Verification items for the finished model (mm, model axes). Face numbers are marked on the shaded views. A direction names the side the tool comes from. Give positions to 0.01 mm unless a question says otherwise; leave off trailing zeros. Order: outer loops, then holes, each group sorted by start corner. A loop starts at its lowest first (then second) coordinate and runs counter-clockwise, first axis right, second up. Notation, with made-up numbers: (65.5, -10.5) - (119.5, -10.5) arc R22 cw to (119.5, -0.5) - close; hole circle Ø11 at (25, -35). An arc over 180 degrees is marked (long way). Answer as a JSON object with one key per item and string values.
```python
from build123d import *

# Parameters (mm, degrees)
SKETCH1_W                    = 22.7711
SKETCH1_H                    = 12.18
BOSS_EXTRUDE1_DEPTH          = 23.79
SKETCH3_W                    = 32.4485
SKETCH3_H                    = 12.18
BOSS_EXTRUDE2_DEPTH          = 2.286
CUT_EXTRUDE1_DEPTH           = 36.695245613
BOSS_EXTRUDE3_DEPTH          = 4.3434
SKETCH6_R                    = 2.3495
BOSS_EXTRUDE4_DEPTH          = 2.7813
SKETCH7_W                    = 2.8956
SKETCH7_H                    = 1.0414
BOSS_EXTRUDE5_DEPTH          = 6.096
M2_5X0_45_TAPPED_HOLE1_D     = 2.05
M2_5X0_45_TAPPED_HOLE1_DEPTH = 4
M2_5X0_45_TAPPED_HOLE1_TIP   = 0.615882135


with BuildPart() as part:
    # Sketch1 → Boss-Extrude1 (new body)
    with BuildSketch(Plane(origin=(0, 0, 0), x_dir=(1, 0, 0), z_dir=(0, 1, 0))):
        with Locations((11.38555, 6.09)):
            Rectangle(SKETCH1_W, SKETCH1_H)
    extrude(amount=BOSS_EXTRUDE1_DEPTH)

    # Sketch3 → Boss-Extrude2 (add)
    with BuildSketch(Plane(origin=(0, 19.0656, 0), x_dir=(1, 0, 0), z_dir=(0, 1, 0))):
        with Locations((11.38555, 6.09)):
            Rectangle(SKETCH3_W, SKETCH3_H)
    extrude(amount=-BOSS_EXTRUDE2_DEPTH)

    # Sketch4 → Cut-Extrude1 (cut, through all)
    with BuildSketch(Plane(origin=(0, 19.0656, 0), x_dir=(1, 0, 0), z_dir=(0, 1, 0))):
        with BuildLine():
            Line((-4.8387, 6.6996), (-3.4671, 6.6996))
            ThreePointArc((-3.4671, 6.6996), (-1.6383, 6.09), (-3.4671, 5.4804))
            Line((-3.4671, 5.4804), (-4.8387, 5.4804))
            Line((-4.8387, 5.4804), (-4.8387, 6.6996))
        make_face()
        with BuildLine():
            Line((26.2382, 5.4804), (27.6098, 5.4804))
            Line((27.6098, 5.4804), (27.6098, 6.6996))
            Line((27.6098, 6.6996), (26.2382, 6.6996))
            ThreePointArc((26.2382, 6.6996), (24.4094, 6.09), (26.2382, 5.4804))
        make_face()
    extrude(amount=-CUT_EXTRUDE1_DEPTH, mode=Mode.SUBTRACT)

    # Sketch5 → Boss-Extrude3 (add)
    with BuildSketch(Plane(origin=(0, 23.79, 0), x_dir=(1, 0, 0), z_dir=(0, 1, 0))):
        with BuildLine():
            ThreePointArc((11.471694537, 8.940519937), (0, 6.09), (11.471694537, 3.239480063))
            ThreePointArc((11.471694537, 3.239480063), (14.5288, 6.09), (11.471694537, 8.940519937))
        make_face()
    extrude(amount=BOSS_EXTRUDE3_DEPTH)

    # Sketch6 → Boss-Extrude4 (add)
    with BuildSketch(Plane(origin=(0, 28.1334, 0), x_dir=(1, 0, 0), z_dir=(0, 1, 0))):
        with Locations(Location((6.09, 6.09, 0), (0, 0, 90))):
            Circle(SKETCH6_R)
    extrude(amount=BOSS_EXTRUDE4_DEPTH)

    # Sketch7 → Boss-Extrude5 (add)
    with BuildSketch(Plane.ZY):
        with Locations((-6.09, 2.3007)):
            Rectangle(SKETCH7_W, SKETCH7_H)
    extrude(amount=BOSS_EXTRUDE5_DEPTH)

    # M2.5x0.45 Tapped Hole1
    with Locations(Plane(origin=(0, 30.9147, 0), x_dir=(1, 0, 0), z_dir=(0, 1, 0))):
        with Locations((6.09, 6.09)):
            Hole(M2_5X0_45_TAPPED_HOLE1_D / 2, depth=M2_5X0_45_TAPPED_HOLE1_DEPTH)
            with Locations((0, 0, -(M2_5X0_45_TAPPED_HOLE1_DEPTH + M2_5X0_45_TAPPED_HOLE1_TIP / 2))):  # 118° drill point
                Cone(0, M2_5X0_45_TAPPED_HOLE1_D / 2, M2_5X0_45_TAPPED_HOLE1_TIP, mode=Mode.SUBTRACT)


solid = part.part
```
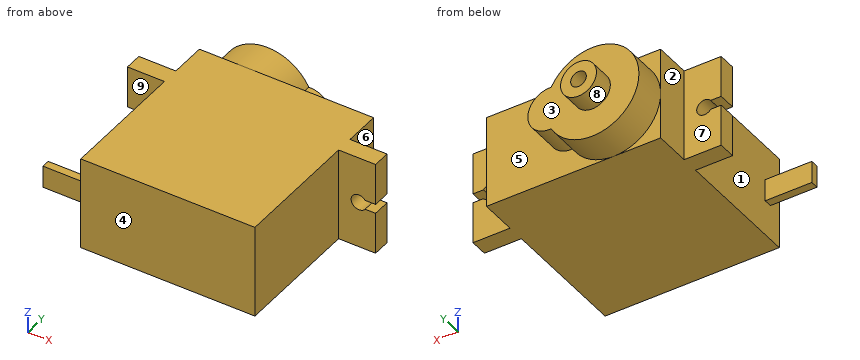
(1) Gauge pin test, flat ends, axial feed: pin 1 Ø1.8 at (x, z) = (6.09, -6.09) entering from +Y; pin 2 Ø0.7 at (y, z) = (18.5, -10.5) entering from -X; pin 3 Ø2.5 at (x, z) = (-2.65, -6.09) entering from -Y; pin 4 Ø1.5 at (x, y) = (-1, 7) entering from -Z. Record the tip position at first contact, or that the pin passes through.
Computed values:
{"pin 1": "stops at y = 26.84", "pin 2": "stops at x = -4.84", "pin 3": "stops at y = 1.78", "pin 4": "passes through"}
(2) Section check B-B (y = 14). Record the cut outline in (x, z), then the cut area to 3 significant figures.
Computed values:
{"outline": "(0, -12.18) - (22.77, -12.18) - (22.77, 0) - (0, 0) - close", "area": "277 mm²"}
(3) Access from +Z, -Z, +X, -X, +Y, -Y to the whole of each face (thin tool, end or side, straight path). Record for the marked faces 5, 6, 7, 8 and 9.
Computed values:
{"face 5": "+X, +Y", "face 6": "+Z, -Z, +X, +Y", "face 7": "+Z, -Z, -X, +Y", "face 8": "+Y", "face 9": "+Z, -Z, -X"}
(4) Section check A-A (z = -10.75). Record the cut outline in (x, y).
Computed values:
{"outline": "(-4.84, 16.78) - (0, 16.78) - (0, 0) - (22.77, 0) - (22.77, 16.78) - (27.61, 16.78) - (27.61, 19.07) - (22.77, 19.07) - (22.77, 23.79) - (10.01, 23.79) - (10.01, 28.13) - (2.17, 28.13) - (2.17, 23.79) - (0, 23.79) - (0, 19.07) - (-4.84, 19.07) - close"}
(5) Release check for a two-part mould opening along Y. For the marked faces 1, 2, 3 and 4 record: pulls with the +Y half, pulls with the -Y half, needs draft (parallel to the pull), parting line crosses it, or undercut.
Computed values:
{"face 1": "undercut", "face 2": "needs draft", "face 3": "pulls with the +Y half", "face 4": "pulls with the -Y half"}
(6) Material ranges on line 1 along X through (y, z) = (29.3, -6.09) (1 decimal); line 2 along Z through (x, y) = (6, 28); line 3 along Y through (x, z) = (14, -5.5), recorded low to high. Write a range as [from, to].
Computed values:
{"line 1": "x = [3.7, 5.1], [7.1, 8.4]", "line 2": "z = [-12.18, -7.11], [-5.07, 0]", "line 3": "y = [0, 28.13]"}
